```python
from build123d import *

# Parameters (mm, degrees)
F0_W     = 13.335
F0_H     = 13.335
F0_R     = 4.3815
F1_DEPTH = 9.652
F2_W     = 0.9652
F2_H     = 13.335
F3_DEPTH = 1.0922
F4_R     = 1.27
F5_R     = 4.8514
F6_DEPTH = 1.0922
F7_W     = 13.335
F7_H     = 4.872686
F8_DEPTH = 0.254


with BuildPart() as f1:
    # F0 (on Top) → F1 (new body)
    with BuildSketch(Plane.XY):
        Rectangle(F0_W, F0_H)
        Circle(F0_R, mode=Mode.SUBTRACT)
    extrude(amount=F1_DEPTH)

    # F2 (on face) → F3 (cut)
    with BuildSketch(Plane.XY.offset(9.652)):
        Rectangle(F2_W, F2_H)
    extrude(amount=-F3_DEPTH, mode=Mode.SUBTRACT)

    # F4
    f4_edges = [f1.edges().sort_by_distance(p)[0] for p in [
        (-6.6675, -6.6675, 4.826),
        (6.6675, -6.6675, 4.826),
        (6.6675, 6.6675, 4.826),
        (-6.6675, 6.6675, 4.826),
    ]]
    fillet(f4_edges, radius=F4_R)

    # F5 (on face) → F6 (cut)
    with BuildSketch(Plane.XY.offset(9.652)):
        Circle(F5_R)
    extrude(amount=-F6_DEPTH, mode=Mode.SUBTRACT)

    # F7 (on face) → F8 (join)
    with BuildSketch(Plane(origin=(0, 0, 0), x_dir=(1, 0, 0), z_dir=(0, 0, -1))):
        with Locations((0, -2.436343)):
            Rectangle(F7_W, F7_H)
    extrude(amount=-F8_DEPTH)


solid = f1.part
```
The listing builds one solid part. Answer for the finished solid, in the listing's coordinates (mm). A direction names the side the tool comes from. Coordinates: 2 decimals unless noted, no trailing zeros. Write each loop counter-clockwise with the first axis right and the second up, starting at its lowest first coordinate (ties: lowest second). Pieces come first, ordered by that corner, then holes. Notation, with made-up numbers: M 40.5,2 L 49.5,2 A26 cw 49.5,27 Z; hole C 88.25,-24.75 d9. An arc over 180 degrees is marked long. Use a Markdown table: item, result. Add a question column.
1. Section B-B (x = 0) is taken. Give the vertices of the cut face in (y, z), plus the area to 3 significant figures.
2. For a pull along X with two mould halves and no side action, classify faces 4 (the flat face through (0, 2, 0)), 5 (the flat face through (0, 2, 0.254)), 6 (the cylindrical face through (-6.305, 6.286, 4.894)) as +X half, -X half, draft (parallel to the pull), parting line (faces both ways), or undercut.
3. Section D-D (x = -3.5) is taken. Give the vertices of the cut face in (y, z).
4. Straight lines are drawn through the part: line 1 along X through (y, z) = (0, 2.75); line 2 along X through (y, z) = (6, 9). For each, find the intervals that lie inside material, in ascending order. Write a range as [from, to].
5. Section C-C (y = -1.75) is taken. Give the vertices of the cut face in (x, z), plus the area to 3 significant figures.
6. Which of the six approach directions +Z, -Z, +X, -X, +Y, -Y give full straight-line access (tool end or side, diameter ignored) to faces 1 (the flat face through (-0.483, -6, 9)), 2 (the flat face through (0, 6.668, 5)), 3 (the cylindrical face through (4.18, 1.32, 4.22))?
7. Section A-A (z = 8) is taken. Give the vertices of the cut face in (x, y), plus the area to 3 significant figures.
8. Given P1, Ø1.5, axis at x = 2, y = -1, coming from the +Z side; P2, Ø3.5, axis at x = -1, y = 2, coming from the +Z side; P3, Ø0.9, axis at y = -6, z = 9.5, coming from the -X side, each flat-ended and moving along its own axis, determine where each tip first touches the part or whether it passes through.
Data:
| question | item | result |
|---|---|---|
| 1 | outline | M -6.67,0 L -4.38,0 L -4.38,8.56 L -6.67,8.56 Z; M 0,0 L 6.67,0 L 6.67,8.56 L 4.38,8.56 L 4.38,0.25 L 0,0.25 Z |
| 1 | area | 40.2 mm2 |
| 2 | face 4 | draft |
| 2 | face 5 | undercut |
| 2 | face 6 | -X half |
| 3 | outline | M -6.67,0 L -2.64,0 L -2.64,8.56 L -3.36,8.56 L -3.36,9.65 L -6.67,9.65 Z; M 0,0 L 6.67,0 L 6.67,9.65 L 3.36,9.65 L 3.36,8.56 L 2.64,8.56 L 2.64,0.25 L 0,0.25 Z |
| 4 | line 1 | x = [-6.67, -4.38], [4.38, 6.67] |
| 4 | line 2 | x = [-6.52, -0.48], [0.48, 6.52] |
| 5 | outline | M -6.67,0 L -4.02,0 L -4.02,8.56 L -4.52,8.56 L -4.52,9.65 L -6.67,9.65 Z; M 4.02,0 L 6.67,0 L 6.67,9.65 L 4.52,9.65 L 4.52,8.56 L 4.02,8.56 Z |
| 5 | area | 50.1 mm2 |
| 6 | face 1 | +Z, +Y, -Y |
| 6 | face 2 | +Z, -Z, +X, -X, +Y |
| 6 | face 3 | +Z |
| 7 | outline | M -6.67,-5.4 A1.27 ccw -5.4,-6.67 L 5.4,-6.67 A1.27 ccw 6.67,-5.4 L 6.67,5.4 A1.27 ccw 5.4,6.67 L -5.4,6.67 A1.27 ccw -6.67,5.4 Z; hole C 0,0 d8.76 |
| 7 | area | 116 mm2 |
| 8 | P1 | passes through |
| 8 | P2 | stops at z = 0.25 |
| 8 | P3 | stops at x = -6.66 |
